from build123d import *

# Parameters (mm, degrees)
BOSS_EXTRUDE1_DEPTH = 2.54
CUT_EXTRUDE2_DEPTH  = 0.254
SKETCH5_R           = 0.482014483
CUT_EXTRUDE3_DEPTH  = 0.508
SKETCH6_R           = 0.508
CUT_EXTRUDE4_DEPTH  = 0.508


with BuildPart() as part:
    # Sketch1 → Boss-Extrude1 (new body)
    with BuildSketch(Plane.XY):
        Polygon((-10.407081712, 5.223554475), (0, 7.738599222), (12.452918288, 4.002723735), (12.452918288, -8.983891051), (0, -12.719766537), (-10.407081712, -10.20472179), (-12.275019455, -10.20472179), (-13.520311284, -10.20472179), (-13.520311284, -8.983891051), (-10.407081712, -8.983891051), (-10.407081712, 4.002723735), (-13.520311284, 4.002723735), (-13.520311284, 5.223554475), (-12.275019455, 5.223554475), align=None)
    extrude(amount=BOSS_EXTRUDE1_DEPTH)

    # Sketch4 → Cut-Extrude2 (cut)
    with BuildSketch(Plane.XY.offset(2.54)):
        Polygon((-9.78623868, 0), (11.923219726, 0), (11.923219726, 2.54), (0, 5.075533386), (-9.78623868, 2.54), align=None)
        Polygon((0, -10.056700701), (-9.78623868, -7.521167315), (-9.78623868, -4.981167315), (11.923219726, -4.981167315), (11.923219726, -7.521167315), align=None)
    extrude(amount=-CUT_EXTRUDE2_DEPTH, mode=Mode.SUBTRACT)

    # Sketch5 → Cut-Extrude3 (cut)
    with BuildSketch(Plane(origin=(0, -8.983891051, 0), x_dir=(1, 0, 0), z_dir=(0, 1, 0))):
        with Locations(Location((-11.963696498, -1.27, 0), (0, 0, 270))):
            Circle(SKETCH5_R)
    extrude(amount=-CUT_EXTRUDE3_DEPTH, mode=Mode.SUBTRACT)

    # Sketch6 → Cut-Extrude4 (cut)
    with BuildSketch(Plane.XZ.offset(-4.002723735)):
        with Locations(Location((-11.963696498, 1.27, 0), (0, 0, 270))):
            Circle(SKETCH6_R)
    extrude(amount=-CUT_EXTRUDE4_DEPTH, mode=Mode.SUBTRACT)


solid = part.part
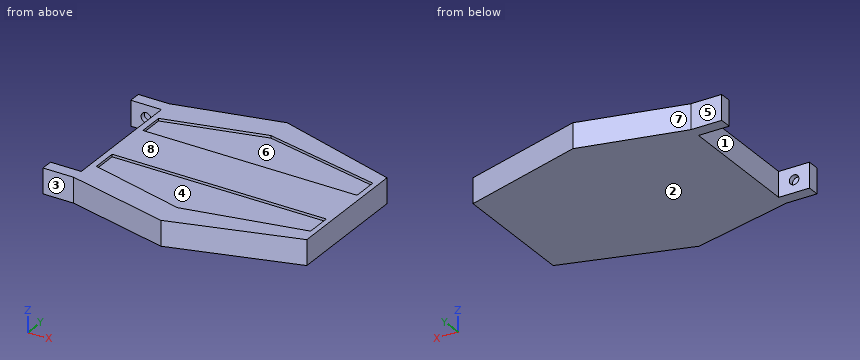
Source: CAD feature listing. Evaluate the final solid. Frame: model axes, mm. Face numbers are marked on the shaded views. A direction names the side the tool comes from. Give positions to 0.01 mm unless a question says otherwise; leave off trailing zeros. Order: outer loops, then holes, each group sorted by start corner. A loop starts at its lowest first (then second) coordinate and runs counter-clockwise, first axis right, second up. Notation, with made-up numbers: (51.25, -29) -> (65.25, -29) arc R18 cw to (65.25, 3) -> close; hole circle Ø4 at (20.25, 77.25). An arc over 180 degrees is marked (long way). Write item = value, one per line.
Q1. Pin query (flat end, axial travel): pin 1 (0.9 mm diameter, centred on x = -11.96, z = 1.27, fed in from +Y); pin 2 (1.1 mm diameter, centred on x = -12, z = 1.5, fed in from -Y); pin 3 (0.8 mm diameter, centred on y = -5, z = 1.5, fed in from -X). Return the tip coordinate at first contact, or that it passes through.
Data:
pin_1 = 5.22
pin_2 = -10.2
pin_3 = -10.41
Q2. Cut plane D-D, the plane y = -4.5. Output: boundary loops of the cut face in (x, z).
Data:
outline = (-10.41, 0) -> (12.45, 0) -> (12.45, 2.54) -> (-10.41, 2.54) -> close
Q3. Material intervals for line 1 (Z direction, x = 9.5, y = -6); line 2 (Y direction, x = -12, z = 2.1); line 3 (X direction, y = -7.5, z = 1.85), sorted ascending. Write a range as from..to.
Data:
line_1 = 0..2.29
line_2 = -10.2..-8.98, 4..5.22
line_3 = -10.41..12.45
Q4. Cut plane A-A, the plane z = 1.27. Output: boundary loops of the cut face in (x, y).
Data:
outline = (-13.52, -10.2) -> (-10.41, -10.2) -> (0, -12.72) -> (12.45, -8.98) -> (12.45, 4) -> (0, 7.74) -> (-10.41, 5.22) -> (-13.52, 5.22) -> (-13.52, 4) -> (-12.47, 4) -> (-12.47, 4.51) -> (-11.46, 4.51) -> (-11.46, 4) -> (-10.41, 4) -> (-10.41, -8.98) -> (-11.48, -8.98) -> (-11.48, -9.49) -> (-12.45, -9.49) -> (-12.45, -8.98) -> (-13.52, -8.98) -> close
Q5. Cut plane C-C, the plane x = -4.75. Output: boundary loops of the cut face in (y, z).
Data:
outline = (-11.57, 0) -> (6.59, 0) -> (6.59, 2.54) -> (3.84, 2.54) -> (3.84, 2.29) -> (0, 2.29) -> (0, 2.54) -> (-4.98, 2.54) -> (-4.98, 2.29) -> (-8.83, 2.29) -> (-8.83, 2.54) -> (-11.57, 2.54) -> close
Q6. Pull-direction query (X, two-part tool) for the marked faces 6, 7 and 8; classes: released by +X, released by -X, zero draft, split by the parting line, or undercut.
Data:
face_6 = undercut
face_7 = released by -X
face_8 = zero draft
Q7. Cut plane B-B, the plane y = 1.5. Output: boundary loops of the cut face in (x, z), and give its area (3 significant figures).
Data:
outline = (-10.41, 0) -> (12.45, 0) -> (12.45, 2.54) -> (11.92, 2.54) -> (11.92, 2.29) -> (-9.79, 2.29) -> (-9.79, 2.54) -> (-10.41, 2.54) -> close
area = 52.6 mm^2
Q8. Set-up query: the marked faces 1, 2, 3, 4 and 5. Return all of +Z, -Z, +X, -X, +Y, -Y with unobstructed straight access to the full face (end or side cutting, diameter ignored); none if empty.
Data:
face_1 = +Z, -Z, -X
face_2 = -Z, +X, -X, +Y, -Y
face_3 = +Z, -Z, -X, -Y
face_4 = +Z
face_5 = +Z, -Z, -X, +Y
